from build123d import *

# Parameters (mm, degrees)
SKETCH_1_R      = 2.75
EXTRUDE_1_DEPTH = 1.5
EXTRUDE_START   = -2.5
SKETCH_2_R      = 2.75
SKETCH_2_R_2    = 1
EXTRUDE_2_DEPTH = 2.5
CHAMFER_1_SIZE  = 0.5


with BuildPart() as part:
    # 스케치1 → 보스-돌출1 (new body)
    with BuildSketch(Plane.XY):
        Circle(SKETCH_1_R)
    extrude(amount=EXTRUDE_1_DEPTH)

    # 스케치2 → 보스-돌출2 (add)
    with BuildSketch(Plane.XY.offset(EXTRUDE_START)):
        Circle(SKETCH_2_R)
        Circle(SKETCH_2_R_2, mode=Mode.SUBTRACT)
    extrude(amount=EXTRUDE_2_DEPTH)

    # 모따기1
    chamfer_1_edges = [part.edges().sort_by_distance(p)[0] for p in [
        (-2.75, 0, 1.5),
        (-2.75, 0, -2.5),
    ]]
    chamfer(chamfer_1_edges, length=CHAMFER_1_SIZE)


solid = part.part
Verification items for the finished model (mm, model axes). A direction names the side the tool comes from. Round coordinates to 2 decimals unless told otherwise and drop trailing zeros. Loops run counter-clockwise (first coordinate to the right, second up) from the corner with the lowest first, then second, coordinate; pieces in that order, holes last. Notation, with made-up numbers: (5, 64.25) - (11, 64.25) arc R16 cw to (11, 76.25) - close; hole circle Ø10 at (-35.5, 34). An arc over 180 degrees is marked (long way). Use one line per item in the form item = value.
1. Section check D-D on z = 0.55. Record the cut outline in (x, y), and give its area (3 significant figures).
A:
outline = circle Ø5.5 at (0, 0)
area = 23.8 mm²
2. Access from +Z, -Z, +X, -X, +Y, -Y to the whole of each face (thin tool, end or side, straight path). Record for faces 4 (the flat face through (-1, -1, -2.5)), 5 (the cylindrical face through (0, -1, -1)).
A:
face_4 = -Z, +X, -X, +Y, -Y
face_5 = -Z
3. Scan lines: probe 1 along Y at (x, z) = (0, -1.8); probe 2 along Y at (x, z) = (-0.65, -0.25); probe 3 along Z at (x, y) = (-0.4, 0.7). Record each from-to range of solid material in increasing order.
A:
probe_1 = -2.75 to -1, 1 to 2.75
probe_2 = -2.67 to -0.76, 0.76 to 2.67
probe_3 = 0 to 1.5
4. Draft check along X on faces 1 (the cylindrical face through (-0.596, -2.685, -0.521)), 2 (the flat face through (0, 0, 0)), 3 (the flat face through (0, 0, 1.5)). Enter one of: pulls with the +X half, pulls with the -X half, needs draft (parallel to the pull), parting line crosses it, or undercut.
A:
face_1 = parting line crosses it
face_2 = undercut
face_3 = needs draft
5. Section check A-A on y = 0. Record the cut outline in (x, z).
A:
outline = (-2.75, -2) - (-2.25, -2.5) - (-1, -2.5) - (-1, 0) - (1, 0) - (1, -2.5) - (2.25, -2.5) - (2.75, -2) - (2.75, 1) - (2.25, 1.5) - (-2.25, 1.5) - (-2.75, 1) - close
6. Gauge pin test, flat ends, axial feed: pin 1 Ø1.6 at (x, y) = (0, 0) entering from -Z; pin 2 Ø2 at (y, z) = (-2, -0.5) entering from -X; pin 3 Ø1 at (y, z) = (-1, -1.5) entering from +X. Record the tip position at first contact, or that the pin passes through.
A:
pin_1 = 0
pin_2 = -2.56
pin_3 = 2.7
7. Section check C-C on z = -0.6. Record the cut outline in (x, y), and give its area (3 significant figures).
A:
outline = circle Ø5.5 at (0, 0); hole circle Ø2 at (0, 0)
area = 20.6 mm²
